Input: part model. Units: mm. Frame: model coordinates. Give positions to 0.01 mm unless a question says otherwise; leave off trailing zeros. Order: outer loops, then holes, each group sorted by start corner. A loop starts at its lowest first (then second) coordinate and runs counter-clockwise, first axis right, second up. Notation, with made-up numbers: M 74,79.5 L 89,79.5 A13 cw 89,95.5 Z; hole C -28,78 d6. An arc over 180 degrees is marked long. Use a Markdown table: item, result.
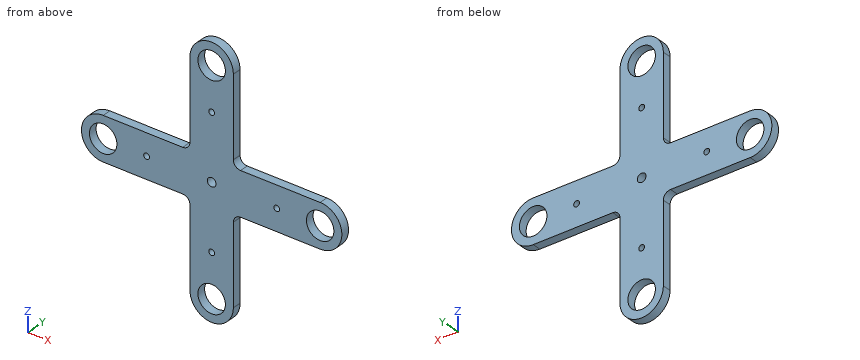
Autodesk Inventor part; units mm, degrees
ref_plane "YZ Plane" through (0, 0, 0) normal (1, 0, 0) x (0, 1, 0)
ref_plane "XZ Plane" through (0, 0, 0) normal (0, 1, 0) x (-1, 0, 0)
ref_plane "XY Plane" through (0, 0, 0) normal (0, 0, 1) x (1, 0, 0)
sketch "Sketch1" plane through (0, 0, 0) normal (0, 1, 0) x (-1, 0, 0)
  circle A0 centre (75, -75) radius 9.5
  arc A1 (75, -90) -> (75, -60) centre (75, -75) ccw
  circle A2 centre (0, 0) radius 9.5
  arc A3 (15, 0) -> (-15, 0) centre (0, 0) ccw
  circle A4 centre (-75, -75) radius 9.5
  arc A5 (-75, -60) -> (-75, -90) centre (-75, -75) ccw
  circle A6 centre (0, -150) radius 9.5
  arc A7 (-15, -150) -> (15, -150) centre (0, -150) ccw
  line L0 (-75, -60) -> (-20, -60)
  line L1 (-75, -90) -> (-20, -90)
  line L2 (75, -60) -> (20, -60)
  line L3 (75, -90) -> (20, -90)
  line L4 (15, 0) -> (15, -55)
  line L5 (15, -95) -> (15, -150)
  line L6 (-15, 0) -> (-15, -55)
  line L7 (-15, -95) -> (-15, -150)
  arc A8 (15, -55) -> (20, -60) centre (20, -55) ccw
  arc A9 (-20, -60) -> (-15, -55) centre (-20, -55) ccw
  arc A10 (20, -90) -> (15, -95) centre (20, -95) ccw
  arc A11 (-15, -95) -> (-20, -90) centre (-20, -95) ccw
  circle A12 centre (0, -30) radius 2
  circle A13 centre (0, -120) radius 2
  circle A14 centre (-45, -75) radius 2
  circle A15 centre (45, -75) radius 2
  circle A16 centre (0, -75) radius 3
  point P0 (15, -60)
  point P1 (15, -90)
  dimension "d5" = 19
  dimension "d6" = 30
  dimension "d7" = 19
  dimension "d8" = 30
  dimension "d9" = 19
  dimension "d10" = 30
  dimension "d11" = 19
  dimension "d12" = 30
  dimension "d13" = 5
  dimension "d15" = 4
  dimension "d17" = 4
  dimension "d19" = 4
  dimension "d21" = 4
  dimension "d22" = 6
extrude "Extrusion1" add sketch "Sketch1" along normal blind 6
properties part number "e_support 1"
1) First-contact query: pin 1 Ø3 at (y, z) = (2, -85) entering from -X; pin 2 Ø1.5 at (y, z) = (3, -112) entering from +X. Flat tips, straight axial feed; report the tip coordinate or a pass-through.
Response values:
| item | result |
|---|---|
| pin 1 | stops at x = -87.36 |
| pin 2 | stops at x = 15 |
2) Cut plane A-A on y = 1.95. State how many separate pieces and enclosed holes the cut face has, and give its area (3 significant figures).
Response values:
| item | result |
|---|---|
| separate pieces | 1 |
| enclosed holes | 9 |
| area | 8,320 mm² |
3) Material intervals for line 1 (Z direction, x = 0, y = 2.5); line 2 (X direction, y = 1.45, z = -69.5); line 3 (Z direction, x = -45, y = 2.7), sorted ascending. Write a range as from..to.
Response values:
| item | result |
|---|---|
| line 1 | z = -165..-159.5, -140.5..-122, -118..-78, -72..-32, -28..-9.5, 9.5..15 |
| line 2 | x = -88.96..-82.75, -67.25..67.25, 82.75..88.96 |
| line 3 | z = -90..-77, -73..-60 |
4) Cut plane B-B on z = -40. Return loops of the section in (x, y).
Response values:
| item | result |
|---|---|
| outline | M -15,0 L 15,0 L 15,6 L -15,6 Z |
5) Cut plane C-C on x = -52. Return loops of the section in (y, z), and give its area (3 significant figures).
Response values:
| item | result |
|---|---|
| outline | M 0,-90 L 6,-90 L 6,-60 L 0,-60 Z |
| area | 180 mm² |
